```python
from build123d import *

# Parameters (mm, degrees)
SKETCH1_W           = 11
SKETCH1_H           = 8
SKETCH1_W_2         = 4
SKETCH1_H_2         = 10
SKETCH1_H_3         = 1
BOSS_EXTRUDE1_DEPTH = 3
SKETCH1_3_W         = 4
SKETCH1_3_H         = 10
BOSS_EXTRUDE2_DEPTH = 8
CUT_EXTRUDE5_DEPTH  = 2.1
HOLE1_D             = 3.2
SKETCH5_W           = 3.4
SKETCH5_H           = 4.5
CUT_EXTRUDE1_DEPTH  = 4
CUT_EXTRUDE4_DEPTH  = 1
SKETCH6_W           = 3.4
SKETCH6_H           = 4.5
CUT_EXTRUDE2_DEPTH  = 2
SKETCH6_3_W         = 3.4
SKETCH6_3_H         = 4.5
CUT_EXTRUDE3_DEPTH  = 32.643953788
FILLET1_R           = 2.5
FILLET2_R           = 2


with BuildPart() as part:
    # Sketch1 → Boss-Extrude1 (new body)
    with BuildSketch(Plane(origin=(0, 0, 0), x_dir=(1, 0, 0), z_dir=(0, 1, 0))):
        with Locations((-32.5, 5)):
            Rectangle(SKETCH1_W, SKETCH1_H)
        Polygon((-23, 10), (-27, 10), (-27, 9), (-27, 1), (-27, 0), (-23, 0), align=None)
        with BuildLine():
            ThreePointArc((-11, 10), (-19, 14.433981132), (-27, 10))
            Line((-27, 10), (-23, 10))
            Line((-23, 10), (-15, 10))
            Line((-15, 10), (-11, 10))
        make_face()
        with Locations((-13, 5)):
            Rectangle(SKETCH1_W_2, SKETCH1_H_2)
        with BuildLine():
            Line((-15, 0), (-23, 0))
            Line((-23, 0), (-27, 0))
            ThreePointArc((-27, 0), (-19, -4.433981132), (-11, 0))
            Line((-11, 0), (-15, 0))
        make_face()
        with Locations((-5.5, 5)):
            Rectangle(SKETCH1_W, SKETCH1_H_2)
        with Locations((-32.5, 9.5)):
            Rectangle(SKETCH1_W, SKETCH1_H_3)
        with Locations((-32.5, 0.5)):
            Rectangle(SKETCH1_W, SKETCH1_H_3)
    extrude(amount=BOSS_EXTRUDE1_DEPTH)

    # Sketch1<3> → Boss-Extrude2 (add)
    with BuildSketch(Plane(origin=(0, 0, 0), x_dir=(1, 0, 0), z_dir=(0, 1, 0))):
        with Locations((-25, 5)):
            Rectangle(SKETCH1_3_W, SKETCH1_3_H)
        with Locations((-13, 5)):
            Rectangle(SKETCH1_3_W, SKETCH1_3_H)
    extrude(amount=-BOSS_EXTRUDE2_DEPTH)

    # Sketch3 → Cut-Extrude5 (cut)
    with BuildSketch(Plane(origin=(0, 3, 0), x_dir=(1, 0, 0), z_dir=(0, 1, 0))):
        Polygon((-7.15, 6.818653348), (-7.15, 3.181346652), (-4, 1.362693304), (-0.85, 3.181346652), (-0.85, 6.818653348), (-4, 8.637306696), align=None)
        Polygon((-30.85, 3.181346652), (-30.85, 6.818653348), (-34, 8.637306696), (-37.15, 6.818653348), (-37.15, 3.181346652), (-34, 1.362693304), align=None)
    extrude(amount=-CUT_EXTRUDE5_DEPTH, mode=Mode.SUBTRACT)

    # Hole1 (through all)
    with Locations(Plane(origin=(-4, 3, -5), x_dir=(0, 0, 1), z_dir=(0, 1, 0))):
        with Locations((0, 0), (0, -30)):
            Hole(HOLE1_D / 2)

    # Sketch5 → Cut-Extrude1 (cut)
    with BuildSketch(Plane.ZY.offset(27)):
        with Locations((-5, -3.75)):
            Rectangle(SKETCH5_W, SKETCH5_H)
    extrude(amount=-CUT_EXTRUDE1_DEPTH, mode=Mode.SUBTRACT)

    # Sketch5<4> → Cut-Extrude4 (cut)
    with BuildSketch(Plane.ZY.offset(27)):
        Polygon((-5, -1.5), (-5, -0.5), (-7.7, -0.5), (-7.7, -7), (-5, -7), (-5, -6), (-6.7, -6), (-6.7, -1.5), align=None)
        Polygon((-2.3, -0.5), (-5, -0.5), (-5, -1.5), (-3.3, -1.5), (-3.3, -6), (-5, -6), (-5, -7), (-2.3, -7), align=None)
    extrude(amount=-CUT_EXTRUDE4_DEPTH, mode=Mode.SUBTRACT)

    # Sketch6 → Cut-Extrude2 (cut)
    # profile 1 of 5: a face of its own
    with BuildSketch(Plane(origin=(-11, 0, 0), x_dir=(0, 0, -1), z_dir=(1, 0, 0))):
        Polygon((3.181346652, -6.3), (6.818653348, -6.3), (8.435234102, -3.5), (6.818653348, -0.7), (3.181346652, -0.7), (1.564765898, -3.5), align=None)
        with Locations((5, -3.75)):
            Rectangle(SKETCH6_W, SKETCH6_H, mode=Mode.SUBTRACT)
    # profile 2 of 5: a face of its own
    with BuildSketch(Plane(origin=(-11, 0, 0), x_dir=(0, 0, -1), z_dir=(1, 0, 0))):
        Polygon((8.435234102, -3.5), (6.818653348, -6.3), (3.181346652, -6.3), (1.564765898, -3.5), (1.362693304, -3.85), (3.181346652, -7), (6.818653348, -7), (8.637306696, -3.85), align=None)
    # profile 3 of 5: a face of its own
    with BuildSketch(Plane(origin=(-11, 0, 0), x_dir=(0, 0, -1), z_dir=(1, 0, 0))):
        Polygon((6.818653348, -0.7), (8.435234102, -3.5), (8.637306696, -3.15), (6.818653348, 0), (3.181346652, 0), (1.362693304, -3.15), (1.564765898, -3.5), (3.181346652, -0.7), align=None)
    # profile 4 of 5: a face of its own
    with BuildSketch(Plane(origin=(-11, 0, 0), x_dir=(0, 0, -1), z_dir=(1, 0, 0))):
        Polygon((8.637306696, -3.15), (8.435234102, -3.5), (8.637306696, -3.85), align=None)
    # profile 5 of 5: a face of its own
    with BuildSketch(Plane(origin=(-11, 0, 0), x_dir=(0, 0, -1), z_dir=(1, 0, 0))):
        Polygon((1.362693304, -3.85), (1.564765898, -3.5), (1.362693304, -3.15), align=None)
    extrude(amount=-CUT_EXTRUDE2_DEPTH, mode=Mode.SUBTRACT)

    # Sketch6<3> → Cut-Extrude3 (cut, through all)
    with BuildSketch(Plane(origin=(-11, 0, 0), x_dir=(0, 0, -1), z_dir=(1, 0, 0))):
        with Locations((5, -3.75)):
            Rectangle(SKETCH6_3_W, SKETCH6_3_H)
    extrude(amount=-CUT_EXTRUDE3_DEPTH, mode=Mode.SUBTRACT)

    # Fillet1
    fillet1_edges = [part.edges().sort_by_distance(p)[0] for p in [
        (-38, 1.5, 0),
        (-38, 1.5, -10),
        (0, 1.5, -10),
        (0, 1.5, 0),
    ]]
    fillet(fillet1_edges, radius=FILLET1_R)

    # Fillet2
    # the kernel refuses this fillet: 2 mm, written as the material it takes off along each edge
    with BuildSketch(Plane(origin=(-11, 0, 0), x_dir=(-1, 0, 0), z_dir=(0, -1, 0)), Plane(origin=(-27, 0, -10), x_dir=(1, 0, 0), z_dir=(0, -1, 0))) as fillet2_piece_1:
        with BuildLine():
            CenterArc((FILLET2_R, FILLET2_R), FILLET2_R, 180, 90)
            Line((0, FILLET2_R), (0, 0))
            Line((0, 0), (FILLET2_R, 0))
        make_face()
    extrude(amount=13, mode=Mode.SUBTRACT)
    with BuildSketch(Plane(origin=(-11, 0, -10), x_dir=(-1, 0, 0), z_dir=(0, -1, 0)), Plane(origin=(-27, 0, 0), x_dir=(1, 0, 0), z_dir=(0, -1, 0))) as fillet2_piece_2:
        with BuildLine():
            CenterArc((FILLET2_R, -FILLET2_R), FILLET2_R, 90, 90)
            Line((0, -FILLET2_R), (0, 0))
            Line((0, 0), (FILLET2_R, 0))
        make_face()
    extrude(amount=13, mode=Mode.SUBTRACT)


solid = part.part
```
CAD build for the part. Positions are in the model's coordinates, mm. A direction names the side the tool comes from. Coordinates: 2 decimals unless noted, no trailing zeros. Order: outer loops, then holes, each group sorted by start corner. A loop starts at its lowest first (then second) coordinate and runs counter-clockwise, first axis right, second up. Notation, with made-up numbers: (66, 12) - (71, 12) arc R24 cw to (71, 49) - close; hole circle Ø2 at (62.25, 27.5). An arc over 180 degrees is marked (long way). Use a Markdown table: item, result. Add a question column.
(1) Which spindle directions (+Z, -Z, +X, -X, +Y, -Y) get a long thin tool onto all of the face, cutting with end or side? Do faces 1 (the face through (-32.447, 1.965, -2.259)), 2 (the face through (-14, -4, 0)), 3 (the face through (-11.986, -5.447, -7.715)). Say none if no direction does.
(2) Drill centre lines: line 1 along X through (y, z) = (0.3, -5); line 2 along Y through (x, z) = (-3, -0.75); line 3 along X through (y, z) = (-3.75, -9). Where is each one in solid material? Low to high. Write a range as [from, to].
(3) Saw through at A-A (y = -7.5). Give the cut face in (x, z).
(4) Pull direction Y, two halves, no side cores. Call faces 4 (the face through (-26.5, -0.5, -5)), 5 (the face through (-30.85, 2, -5)): +Y half, -Y half, draft (parallel to the pull), parting line (faces both ways), or undercut.
(5) Flat gauge pins, fed straight in: pin 1 (1.5 mm diameter, centred on y = -4.5, z = -6.5, fed in from -X); pin 2 (5 mm diameter, centred on y = -5, z = 2, fed in from -X); pin 3 (1.6 mm diameter, centred on x = -14, y = -2.5, fed in from -Z). Where does each tip first touch, or does it go through?
(6) Saw through at C-C (y = -2.5). Give the cut face in (x, z), then the cut area to 3 significant figures.
(7) Saw through at B-B (x = -22.5). Give the cut face in (y, z), then the cut area to 3 significant figures.
(8) Saw through at D-D (z = -0.75). Give the cut face in (x, y).
Solved:
| question | item | result |
|---|---|---|
| 1 | face 1 | +Y |
| 1 | face 2 | +Z, +X, -X, -Y |
| 1 | face 3 | +X |
| 2 | line 1 | x = [-38, -35.6], [-32.4, -23], [-15, -5.6], [-2.4, 0] |
| 2 | line 2 | y = [0, 3] |
| 2 | line 3 | x = [-26.73, -23], [-15, -11.27] |
| 3 | outline | (-27, -8) arc R2 ccw to (-25, -10) - (-23, -10) - (-23, 0) - (-25, 0) arc R2 ccw to (-27, -2) - close; (-15, -10) - (-13, -10) arc R2 ccw to (-11, -8) - (-11, -2) arc R2 ccw to (-13, 0) - (-15, 0) - close |
| 4 | face 4 | undercut |
| 4 | face 5 | draft |
| 5 | pin 1 | stops at x = -26 |
| 5 | pin 2 | stops at x = -26.32 |
| 5 | pin 3 | stops at z = -10 |
| 6 | outline | (-27, -8) arc R2 ccw to (-25, -10) - (-23, -10) - (-23, -6.7) - (-26, -6.7) - (-26, -7.7) - (-27, -7.7) - close; (-27, -2.3) - (-26, -2.3) - (-26, -3.3) - (-23, -3.3) - (-23, 0) - (-25, 0) arc R2 ccw to (-27, -2) - close; (-15, -10) - (-13, -10) arc R2 ccw to (-11.02, -8.26) - (-13, -8.26) - (-13, -6.7) - (-15, -6.7) - close; (-15, -3.3) - (-13, -3.3) - (-13, -1.74) - (-11.02, -1.74) arc R2 ccw to (-13, 0) - (-15, 0) - close |
| 6 | area | 41.1 mm² |
| 7 | outline | (0, -13.76) - (3, -13.76) - (3, -10) - (0, -10) - close; (0, 0) - (3, 0) - (3, 3.76) - (0, 3.76) - close |
| 7 | area | 22.6 mm² |
| 8 | outline | (-37.29, 0) - (-26.56, 0) - (-26.56, -8) - (-23, -8) - (-23, 3) - (-37.29, 3) - close; (-15, -8) - (-11.44, -8) - (-11.44, 0) - (-0.71, 0) - (-0.71, 3) - (-15, 3) - close |
